from build123d import *

# Parameters (mm, degrees)
ESBO_O1_W                     = 45
ESBO_O1_H                     = 10
RESSALTO_EXTRUS_O1_DEPTH      = 55
RESSALTO_EXTRUS_O2_DEPTH      = 100
RESSALTO_EXTRUS_O2_DEPTH_BACK = 20
ESBO_O2_W                     = 90
ESBO_O2_H                     = 5
RESSALTO_EXTRUS_O3_DEPTH      = 5
FILETE1_R                     = 20
ESBO_O6_R                     = 1.5
CORTE_EXTRUS_O1_DEPTH         = 10


with BuildPart() as part:
    # Esboço1 → Ressalto-extrusão1 (new body)
    with BuildSketch(Plane.XY):
        Rectangle(ESBO_O1_W, ESBO_O1_H)
    extrude(amount=RESSALTO_EXTRUS_O1_DEPTH)

    # Esboço2 → Ressalto-extrusão2 (add, two sides: drawn at the far end of the back side and taken through both)
    with BuildSketch(Plane(origin=(0, 5, 0), x_dir=(1, 0, 0), z_dir=(0, 1, 0)).offset(-RESSALTO_EXTRUS_O2_DEPTH_BACK)):
        with Locations((0, -57.5)):
            Rectangle(ESBO_O2_W, ESBO_O2_H)
    extrude(amount=RESSALTO_EXTRUS_O2_DEPTH + RESSALTO_EXTRUS_O2_DEPTH_BACK)

    # Esboço5 → Ressalto-extrusão3 (add)
    with BuildSketch(Plane(origin=(22.5, 0, 0), x_dir=(0, 0, -1), z_dir=(1, 0, 0))):
        Polygon((-55, -5), (0, -5), (-55, -15), align=None)
    ressalto_extrus_o3 = extrude(amount=-RESSALTO_EXTRUS_O3_DEPTH)

    # Espelhar1: Ressalto-extrusão3 across plane
    add(ressalto_extrus_o3.mirror(Plane(origin=(0, 0, 0), x_dir=(0, 0, 1), z_dir=(1, 0, 0))))

    # Filete1
    filete1_edges = [part.edges().sort_by_distance(p)[0] for p in [
        (-22.5, -5, 55),
        (22.5, -5, 55),
        (0, 5, 55),
    ]]
    fillet(filete1_edges, radius=FILETE1_R)

    # Esboço6 → Corte-extrusão1 (cut)
    with BuildSketch(Plane(origin=(0, 0, 0), x_dir=(-1, 0, 0), z_dir=(0, 0, -1))):
        with Locations((-17.673330857, 0)):
            Circle(ESBO_O6_R)
        with Locations((17.326669143, 0)):
            Circle(ESBO_O6_R)
    extrude(amount=-CORTE_EXTRUS_O1_DEPTH, mode=Mode.SUBTRACT)


solid = part.part
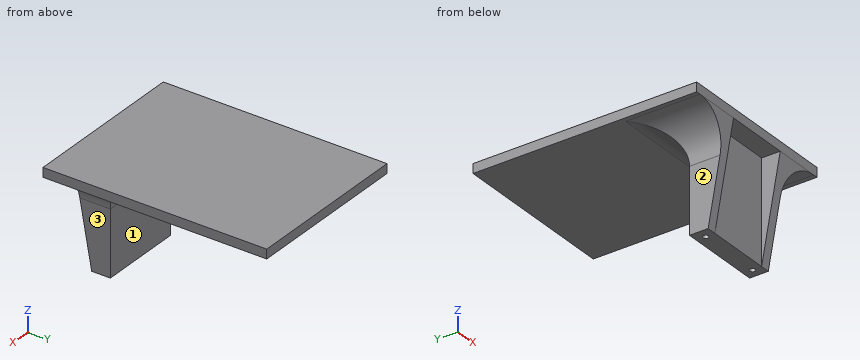
Design review of the part built by this model. Coordinates are the model's own, in mm. Face numbers are marked on the shaded views. A direction names the side the tool comes from. Round coordinates to 2 decimals unless told otherwise and drop trailing zeros. Write each loop counter-clockwise with the first axis right and the second up, starting at its lowest first coordinate (ties: lowest second). Pieces come first, ordered by that corner, then holes. Notation, with made-up numbers: (-11, 78) - (7, 78) arc R18 cw to (7, 84) - close; hole circle Ø1 at (-37, -23.75). An arc over 180 degrees is marked (long way). Return JSON: item names as keys, results as strings. Group by question number.
Item 1: We need section B-B on x = -20.5. Write out the cut boundary in (y, z).
Item 2: Machinability: for the marked faces 1, 2 and 3, which of the approach directions +Z, -Z, +X, -X, +Y, -Y give a long, thin tool a straight path to every point of the face, cutting with its end or side? Answer none if there is none.
Item 3: Insertion check: P1, Ø10.5, axis at x = -3.5, z = 39.5, coming from the -Y side; P2, Ø8, axis at y = -7.5, z = 15.5, coming from the -X side; P3, Ø18, axis at y = -2, z = 12.5, coming from the +X side. Each pin has a flat end and moves straight along its axis. Give the tip position at first contact, or say it passes through.
Item 4: We need section C-C on z = 6. Write out the cut boundary in (x, y).
Item 5: For probe 1 along Z at (x, y) = (-13, 30); probe 2 along Y at (x, z) = (-16.5, 32); probe 3 along Y at (x, z) = (19, 5), list the stretches that pass through material, from the lowest coordinate up. Write a range as [from, to].
Item 6: We need section A-A on y = 0. Write out the cut boundary in (x, z), and give its area (3 significant figures).
Item 7: We need section D-D on z = 38. Write out the cut boundary in (x, y).
Model answer:
{
 "1": {"outline": "(-15, 55) - (-5, 0) - (5, 0) - (5, 35) arc R20 cw to (25, 55) - (105, 55) - (105, 60) - (-15, 60) - close"},
 "2": {"face 1": "-Z, +X, -X, +Y", "face 2": "-Z, -X, +Y, -Y", "face 3": "-Z, +X, +Y, -Y"},
 "3": {"P1": "stops at y = -5", "P2": "stops at x = -22.5", "P3": "stops at x = 22.5"},
 "4": {"outline": "(-22.5, -6.09) - (-17.5, -6.09) - (-17.5, -5) - (17.5, -5) - (17.5, -6.09) - (22.5, -6.09) - (22.5, 5) - (-22.5, 5) - close; hole circle Ø3 at (-17.33, 0); hole circle Ø3 at (17.67, 0)"},
 "5": {"probe 1": "z = [55, 60]", "probe 2": "y = [-5, 5]", "probe 3": "y = [-5.91, -0.7], [0.7, 5]"},
 "6": {"outline": "(-45, 55) - (-42.5, 55) arc R20 cw to (-22.5, 35) - (-22.5, 0) - (-18.83, 0) - (-18.83, 10) - (-15.83, 10) - (-15.83, 0) - (16.17, 0) - (16.17, 10) - (19.17, 10) - (19.17, 0) - (22.5, 0) - (22.5, 35) arc R20 cw to (42.5, 55) - (45, 55) - (45, 60) - (-45, 60) - close", "area": "3,040 mm²"},
 "7": {"outline": "(-22.73, -11.91) - (-17.5, -11.91) - (-17.5, -5) - (17.5, -5) - (17.5, -11.91) - (22.73, -11.91) - (22.73, 5.23) - (-22.73, 5.23) - close"}
}
